```python
from build123d import *

# Parameters (mm, degrees)
ESBO_O1_W                  = 71.15
ESBO_O1_H                  = 72
RESSALTO_EXTRUS_O1_DEPTH   = 1.5
ESBO_O2_W                  = 71.15
ESBO_O2_H                  = 72
ESBO_O2_W_2                = 67.15
ESBO_O2_H_2                = 68
RESSALTO_EXTRUS_O2_DEPTH   = 22
FILETE1_R                  = 2
ESBO_O3_W                  = 13
ESBO_O3_H                  = 25
CORTE_EXTRUS_O1_DEPTH      = 20
RESSALTO_EXTRUS_O3_DEPTH   = 6
ESBO_O5_W                  = 9
ESBO_O5_H                  = 11
CORTE_EXTRUS_O2_DEPTH      = 1
CORTE_EXTRUS_O2_DEPTH_BACK = 2
ESBO_O6_W                  = 8.5
ESBO_O6_H                  = 12
CORTE_EXTRUS_O3_DEPTH      = 2
ESBO_O7_W                  = 7.5
ESBO_O7_H                  = 7.5
RESSALTO_EXTRUS_O4_DEPTH   = 6
ESBO_O8_W                  = 6
ESBO_O8_H                  = 6
RESSALTO_EXTRUS_O5_DEPTH   = 6
RESSALTO_EXTRUS_O6_DEPTH   = 7
ESBO_O10_W                 = 25.22
ESBO_O10_H                 = 13.22
CORTE_EXTRUS_O4_DEPTH      = 3
FILETE3_R                  = 1
FILETE4_R                  = 1


with BuildPart() as part:
    # Esboço1 → Ressalto-extrusão1 (new body, symmetric)
    with BuildSketch(Plane(origin=(0, 0, 0), x_dir=(1, 0, 0), z_dir=(0, 1, 0))):
        Rectangle(ESBO_O1_W, ESBO_O1_H)
    extrude(amount=RESSALTO_EXTRUS_O1_DEPTH, both=True)

    # Esboço2 → Ressalto-extrusão2 (add)
    with BuildSketch(Plane(origin=(0, 1.5, 0), x_dir=(1, 0, 0), z_dir=(0, 1, 0))):
        Rectangle(ESBO_O2_W, ESBO_O2_H)
        Rectangle(ESBO_O2_W_2, ESBO_O2_H_2, mode=Mode.SUBTRACT)
    extrude(amount=RESSALTO_EXTRUS_O2_DEPTH)

    # Filete1
    filete1_edges = [part.edges().sort_by_distance(p)[0] for p in [
        (-33.575, 12.5, -34),
        (-33.575, 12.5, 34),
        (33.575, 12.5, 34),
        (33.575, 12.5, -34),
        (-35.575, 11, -36),
        (35.575, 11, -36),
        (35.575, 11, 36),
        (-35.575, 11, 36),
    ]]
    fillet(filete1_edges, radius=FILETE1_R)

    # Esboço3 → Corte-extrusão1 (cut)
    with BuildSketch(Plane(origin=(0, 0, -36), x_dir=(-1, 0, 0), z_dir=(0, 0, -1))):
        with Locations((-9.375, 11)):
            Rectangle(ESBO_O3_W, ESBO_O3_H)
    extrude(amount=-CORTE_EXTRUS_O1_DEPTH, mode=Mode.SUBTRACT)

    # Esboço4 → Ressalto-extrusão3 (add)
    with BuildSketch(Plane(origin=(0, 1.5, 0), x_dir=(1, 0, 0), z_dir=(0, 1, 0))):
        Polygon((17.875, 34), (17.875, 14), (0.875, 14), (0.875, 34), (2.875, 34), (2.875, 16), (15.875, 16), (15.875, 34), align=None)
    extrude(amount=RESSALTO_EXTRUS_O3_DEPTH)

    # Esboço5 → Corte-extrusão2 (cut, two sides)
    with BuildSketch(Plane(origin=(35.575, 0, 0), x_dir=(0, 0, -1), z_dir=(1, 0, 0))) as corte_extrus_o2_sk:
        with Locations((-13, 18)):
            Rectangle(ESBO_O5_W, ESBO_O5_H)
    extrude(amount=CORTE_EXTRUS_O2_DEPTH, mode=Mode.SUBTRACT)
    extrude(corte_extrus_o2_sk.sketch, amount=-CORTE_EXTRUS_O2_DEPTH_BACK, mode=Mode.SUBTRACT)

    # Esboço6 → Corte-extrusão3 (cut)
    with BuildSketch(Plane(origin=(35.575, 0, 0), x_dir=(0, 0, -1), z_dir=(1, 0, 0))):
        with Locations((-2.25, 17.5)):
            Rectangle(ESBO_O6_W, ESBO_O6_H)
    extrude(amount=-CORTE_EXTRUS_O3_DEPTH, mode=Mode.SUBTRACT)

    # Esboço7 → Ressalto-extrusão4 (add)
    with BuildSketch(Plane(origin=(0, 1.5, 0), x_dir=(1, 0, 0), z_dir=(0, 1, 0))):
        with Locations((-27.075, -25)):
            Rectangle(ESBO_O7_W, ESBO_O7_H)
        Polygon((-28.66271324, -22.25), (-30.250426481, -25), (-28.66271324, -27.75), (-25.48728676, -27.75), (-23.899573519, -25), (-25.48728676, -22.25), align=None, mode=Mode.SUBTRACT)
        with Locations((19.875, -25)):
            Rectangle(ESBO_O7_W, ESBO_O7_H)
        Polygon((18.28728676, -22.25), (16.699573519, -25), (18.28728676, -27.75), (21.46271324, -27.75), (23.050426481, -25), (21.46271324, -22.25), align=None, mode=Mode.SUBTRACT)
        with Locations((19.875, -0.5)):
            Rectangle(ESBO_O7_W, ESBO_O7_H)
        Polygon((21.46271324, -3.25), (18.28728676, -3.25), (16.699573519, -0.5), (18.28728676, 2.25), (21.46271324, 2.25), (23.050426481, -0.5), align=None, mode=Mode.SUBTRACT)
        with Locations((-27.075, -0.5)):
            Rectangle(ESBO_O7_W, ESBO_O7_H)
        Polygon((-25.48728676, -3.25), (-28.66271324, -3.25), (-30.250426481, -0.5), (-28.66271324, 2.25), (-25.48728676, 2.25), (-23.899573519, -0.5), align=None, mode=Mode.SUBTRACT)
    extrude(amount=RESSALTO_EXTRUS_O4_DEPTH)

    # Esboço8 → Ressalto-extrusão5 (add)
    with BuildSketch(Plane(origin=(0, 1.5, 0), x_dir=(1, 0, 0), z_dir=(0, 1, 0))):
        with Locations((-26.825, 24.9)):
            Rectangle(ESBO_O8_W, ESBO_O8_H)
        Polygon((-27.979700538, 26.9), (-29.134401077, 24.9), (-27.979700538, 22.9), (-25.670299462, 22.9), (-24.515598923, 24.9), (-25.670299462, 26.9), align=None, mode=Mode.SUBTRACT)
        with Locations((-1.605, 24.9)):
            Rectangle(ESBO_O8_W, ESBO_O8_H)
        Polygon((-2.759700538, 26.9), (-3.914401077, 24.9), (-2.759700538, 22.9), (-0.450299462, 22.9), (0.704401077, 24.9), (-0.450299462, 26.9), align=None, mode=Mode.SUBTRACT)
        with Locations((-1.605, 5.68)):
            Rectangle(ESBO_O8_W, ESBO_O8_H)
        Polygon((-2.759700538, 7.68), (-3.914401077, 5.68), (-2.759700538, 3.68), (-0.450299462, 3.68), (0.704401077, 5.68), (-0.450299462, 7.68), align=None, mode=Mode.SUBTRACT)
        with Locations((-26.825, 5.68)):
            Rectangle(ESBO_O8_W, ESBO_O8_H)
        Polygon((-27.979700538, 7.68), (-29.134401077, 5.68), (-27.979700538, 3.68), (-25.670299462, 3.68), (-24.515598923, 5.68), (-25.670299462, 7.68), align=None, mode=Mode.SUBTRACT)
    extrude(amount=RESSALTO_EXTRUS_O5_DEPTH)

    # Esboço9 → Ressalto-extrusão6 (add)
    with BuildSketch(Plane(origin=(0, 1.5, 0), x_dir=(1, 0, 0), z_dir=(0, 1, 0))):
        Polygon((-23.825, 22.9), (-4.605, 22.9), (0.895, 22.9), (0.895, 7.68), (-4.605, 7.68), (-23.825, 7.68), (-26.325, 7.68), (-26.325, 22.9), align=None)
        Polygon((-23.825, 21.9), (-4.605, 21.9), (-0.105, 21.9), (-0.105, 8.68), (-4.605, 8.68), (-23.825, 8.68), (-25.325, 8.68), (-25.325, 21.9), align=None, mode=Mode.SUBTRACT)
    extrude(amount=RESSALTO_EXTRUS_O6_DEPTH)

    # Esboço10 → Corte-extrusão4 (cut)
    with BuildSketch(Plane(origin=(0, 1.5, 0), x_dir=(1, 0, 0), z_dir=(0, 1, 0))):
        with Locations((-12.715, 15.29)):
            Rectangle(ESBO_O10_W, ESBO_O10_H)
    extrude(amount=-CORTE_EXTRUS_O4_DEPTH, mode=Mode.SUBTRACT)

    # Filete3
    filete3_edges = [part.edges().sort_by_distance(p)[0] for p in [
        (-25.325, 3.5, -8.68),
        (-25.325, 3.5, -21.9),
        (-0.105, 3.5, -8.68),
        (-0.105, 3.5, -21.9),
        (-12.715, -1.5, -21.9),
        (-0.105, -1.5, -15.29),
        (-12.715, -1.5, -8.68),
        (-25.325, -1.5, -15.29),
    ]]
    fillet(filete3_edges, radius=FILETE3_R)

    # Filete4
    filete4_edges = [part.edges().sort_by_distance(p)[0] for p in [
        (2.875, -1.5, -26),
        (-15.35, -1.5, -36),
        (-34.989213562, -1.5, -35.414213562),
        (-35.575, -1.5, 0),
        (-34.989213562, -1.5, 35.414213562),
        (0, -1.5, 36),
        (34.989213562, -1.5, 35.414213562),
        (35.575, -1.5, 0),
        (34.989213562, -1.5, -35.414213562),
        (24.725, -1.5, -36),
        (15.875, -1.5, -26),
        (9.375, -1.5, -16),
        (35.575, 18, 17.5),
        (35.575, 12.5, 13),
        (35.575, 11.5, 2.25),
        (35.575, 17.5, -2),
        (15.875, 11, -36),
        (2.875, 11, -36),
    ]]
    fillet(filete4_edges, radius=FILETE4_R)


solid = part.part
```
For this review, take the finished solid that the model builds, in its own axes (mm). Round coordinates to 2 decimals unless told otherwise and drop trailing zeros. Write each loop counter-clockwise with the first axis right and the second up, starting at its lowest first coordinate (ties: lowest second). Pieces come first, ordered by that corner, then holes. Notation, with made-up numbers: (-31.75, -27) - (-17.75, -27) arc R25 cw to (-17.75, 1) - close; hole circle Ø1 at (44.5, 46.25). An arc over 180 degrees is marked (long way). Put each result on its own line as item: value.
Q1. Mouldability with a two-part tool opening along Z and no side actions: class faces 1 (the face through (0.135, 4.458, -6.666)), 2 (the face through (0, 11, 36)) as released by +Z, released by -Z, zero draft, split by the parting line, or undercut.
Solved:
face 1: undercut
face 2: released by +Z
Q2. We need section A-A (x = -6.5). Give the boundary of the cut face in (y, z), and give its area (3 significant figures).
Solved:
outline: (-1.5, -35) arc R1 ccw to (-0.5, -36) - (23.5, -36) - (23.5, -34) - (1.5, -34) - (1.5, -22.9) - (8.5, -22.9) - (8.5, -21.9) - (-0.5, -21.9) arc R1 ccw to (-1.5, -22.9) - close; (-1.5, -7.68) arc R1 ccw to (-0.5, -8.68) - (8.5, -8.68) - (8.5, -7.68) - (1.5, -7.68) - (1.5, 34) - (23.5, 34) - (23.5, 36) - (-0.5, 36) arc R1 ccw to (-1.5, 35) - close
area: 277 mm2
Q3. We need section D-D (x = 5.5). Give the boundary of the cut face in (y, z), and give its area (3 significant figures).
Solved:
outline: (-1.5, -15) arc R1 ccw to (-0.5, -16) - (7.5, -16) - (7.5, -14) - (1.5, -14) - (1.5, 34) - (23.5, 34) - (23.5, 36) - (-0.5, 36) arc R1 ccw to (-1.5, 35) - close
area: 212 mm2
Q4. We need section B-B (y = 20.75). Count the separate pieces of the cut face and the enclosed holes in it, and give its area (3 significant figures).
Solved:
separate pieces: 3
enclosed holes: 0
area: 495 mm2
Q5. We need section C-C (z = 9.5). Give the boundary of the cut face in (x, y) (3 decimals), and give its area (3 significant figures).
Solved:
outline: (-35.575, -0.5) arc R1 ccw to (-34.575, -1.5) - (34.575, -1.5) arc R1 ccw to (35.575, -0.5) - (35.575, 11.5) arc R1 ccw to (34.575, 12.5) - (33.575, 12.5) - (33.575, 1.5) - (-33.575, 1.5) - (-33.575, 23.5) - (-35.575, 23.5) - close
area: 279 mm2
Q6. Insertion check: pin 1 Ø6 at (x, z) = (-10, 23.5) entering from +Y; pin 2 Ø1.5 at (x, z) = (0.5, -28.5) entering from +Y; pin 3 Ø4.5 at (x, z) = (-2.5, -24.5) entering from +Y. Each pin has a flat end and moves straight along its axis. Give the tip position at first contact, or say it passes through.
Solved:
pin 1: stops at y = 1.5
pin 2: stops at y = 7.5
pin 3: stops at y = 8.5
Q7. Wall thickness on probe 1 along X at (y, z) = (3.5, -19) (3 decimals); probe 2 along Z at (x, y) = (-7, 17.75); probe 3 along X at (y, z) = (14.5, -13.5) (3 decimals): over which ranges is each line inside the solid? List them lowest first.
Solved:
probe 1: x = -35.575 to -33.575, -26.325 to -25.325, -0.105 to 2.875, 15.875 to 17.875, 33.575 to 35.575
probe 2: z = -36 to -34, 34 to 36
probe 3: x = -35.575 to -33.575, 33.575 to 35.575
